The model under review builds one solid part; all positions refer to its coordinate system, in mm. A direction names the side the tool comes from. Coordinates: 2 decimals unless noted, no trailing zeros. Order: outer loops, then holes, each group sorted by start corner. A loop starts at its lowest first (then second) coordinate and runs counter-clockwise, first axis right, second up. Notation, with made-up numbers: M 53.5,-22.5 L 103.5,-22.5 A29 ccw 103.5,5.5 Z; hole C 87.25,68.25 d10. An arc over 180 degrees is marked long. Write each question's results on one line, items separated by ' | '.
from build123d import *

# Parameters (mm, degrees)
F1_DEPTH    = 1.5
F2_R        = 1.4
F3_DEPTH    = 4
F4_R        = 1.7145
F5_DEPTH    = 2
F6_SIZE     = 0.4572
F7_S5_R     = 1.4
F7_T6_DEPTH = 4
F8_R        = 3
F9_DEPTH    = 2
F10_DEPTH   = 25.4


# Not quite as in the source:
# - a fillet or chamfer that OpenCascade refuses, or shapes differently, is made with other operations: its cross-section is extruded or revolved along the edge and cut away or added


with BuildPart() as f1:
    # F0 (on Top) → F1 (new body)
    with BuildSketch(Plane.XY):
        with BuildLine():
            Line((-9.5, -3), (7, -3))
            ThreePointArc((7, -3), (4, 0), (7, 3))
            Line((7, 3), (-9.5, 3))
            ThreePointArc((-9.5, 3), (-7.3786796564, 2.1213203436), (-6.5, 0))
            ThreePointArc((-6.5, 0), (-7.3786796564, -2.1213203436), (-9.5, -3))
        make_face()
        with BuildLine():
            ThreePointArc((7, 3), (4, 0), (7, -3))
            ThreePointArc((7, -3), (9.1213203436, -2.1213203436), (10, 0))
            ThreePointArc((10, 0), (9.1213203436, 2.1213203436), (7, 3))
        make_face()
        with BuildLine():
            ThreePointArc((-9.5, 3), (-12.5, 0), (-9.5, -3))
            Line((-9.5, -3), (-9.5, -1.5))
            ThreePointArc((-9.5, -1.5), (-11, 0), (-9.5, 1.5))
            Line((-9.5, 1.5), (-9.5, 3))
        make_face()
        with BuildLine():
            Line((-9.5, -1.5), (-9.5, -3))
            ThreePointArc((-9.5, -3), (-7.3786796564, -2.1213203436), (-6.5, 0))
            ThreePointArc((-6.5, 0), (-7.3786796564, 2.1213203436), (-9.5, 3))
            Line((-9.5, 3), (-9.5, 1.5))
            ThreePointArc((-9.5, 1.5), (-8.4393398282, 1.0606601718), (-8, 0))
            ThreePointArc((-8, 0), (-8.4393398282, -1.0606601718), (-9.5, -1.5))
        make_face()
    extrude(amount=F1_DEPTH)

    # F2 (on face) → F3 (join)
    with BuildSketch(Plane.XY.offset(1.5)):
        with Locations((7, 0)):
            Circle(F2_R)
    extrude(amount=F3_DEPTH)

    # F4 (on face) → F5 (join)
    with BuildSketch(Plane.XY.offset(5.5)):
        with Locations((7, 0)):
            Circle(F4_R)
    extrude(amount=-F5_DEPTH)

    # F6
    f6_edges = [f1.edges().sort_by_distance(p)[0] for p in [
        (5.2855, 0, 5.5),
    ]]
    chamfer(f6_edges, length=F6_SIZE)

    # F7: chamfer of 0.4572 on 1 edges, made by hand


with BuildPart() as f7_tool2:
    # F7_s3 → F7_t4 (revolve)
    with BuildSketch(Plane.XZ):
        Polygon((8.7145, 3.9572), (8.2573, 3.5), (8.7145, 3.5), align=None)
    revolve(axis=Axis((7, 0, 3.5), (0, 0, 1)))

    # F7_s5 → F7_t6 (cut, symmetric)
    with BuildSketch(Plane.XY.offset(3.7)):
        with Locations((7, 0)):
            Circle(F7_S5_R)
    extrude(amount=F7_T6_DEPTH, both=True, mode=Mode.SUBTRACT)


with BuildPart() as f1_1:
    add(f1.part)

    # F7_t1: cut F7_tool2
    add(f7_tool2.part, mode=Mode.SUBTRACT)

    # F8 (on face) → F9 (join)
    with BuildSketch(Plane.XY.offset(1.5)):
        with Locations((-9.5, 0)):
            Circle(F8_R)
    extrude(amount=F9_DEPTH)

    # F10 (cut): a face of the model
    f10_faces = [f1_1.faces().sort_by_distance(p)[0] for p in [
        (-9.5, 0, 1.5),
    ]]
    extrude(f10_faces, amount=-F10_DEPTH, mode=Mode.SUBTRACT)


solid = f1_1.part
1) For faces 5 (the cylindrical face through (5.287, 0.075, 4.508)), 6 (the cylindrical face through (5.6, 0.06, 2.59)), 7 (the flat face through (-11, -1, 3.5)), list the 3-axis set-ups (+Z, -Z, +X, -X, +Y, -Y) from which the entire face can be reached by the end or side of a thin tool; tool diameter is ignored.
Solutions:
face 5: +Z | face 6: none | face 7: +Z, -X, +Y, -Y
2) The part is to be moulded in two halves that separate along Y. For faces 1 (the cylindrical face through (-12.5, 0.1, 2.1)), 2 (the flat face through (7, 0, 5.5)), 3 (the flat face through (-1, 3, 1)), 4 (the cylindrical face through (-8, 0, 2)), say which applies: pulls with the +Y half, pulls with the -Y half, needs draft (parallel to the pull), parting line crosses it, or undercut.
Solutions:
face 1: parting line crosses it | face 2: needs draft | face 3: pulls with the +Y half | face 4: undercut
3) Take a section at B-B on x = 0. State the section outline as (y, z) points, plus the area to 3 significant figures.
Solutions:
outline: M -3,0 L 3,0 L 3,1.5 L -3,1.5 Z | area: 9.00 mm2
4) Take a section at A-A on z = 2.9. State the section outline as (x, y) points, plus the area to 3 significant figures.
Solutions:
outline: C -9.5,0 d6; C 7,0 d2.8; hole C -9.5,0 d3 | area: 27.4 mm2
5) To check wall thickness, follow line 1 along Y through (x, z) = (-9.5, 1.9); line 2 along Z through (x, y) = (-9.25, 2.05); line 3 along Z through (x, y) = (1.5, 1.85). State the ranges of each line that lie inside material, in increasing order.
Solutions:
line 1: -3 to -1.5, 1.5 to 3 | line 2: 0 to 3.5 | line 3: 0 to 1.5
6) Take a section at C-C on z = 4.2. State the section outline as (x, y) points.
Solutions:
outline: C 7,0 d3.43
